Autodesk Inventor part; units mm, degrees
ref_plane "YZ Plane" through (0, 0, 0) normal (1, 0, 0) x (0, 1, 0)
ref_plane "XZ Plane" through (0, 0, 0) normal (0, 1, 0) x (-1, 0, 0)
ref_plane "XY Plane" through (0, 0, 0) normal (0, 0, 1) x (1, 0, 0)
sketch "Sketch1" plane through (0, 0, 0) normal (0, 0, 1) x (1, 0, 0)
  line L0 (0, 50.2073) -> (47.75, 15.5149) construction
  line L1 (47.75, 15.5149) -> (29.5111, -40.6186) construction
  line L2 (29.5111, -40.6186) -> (-29.5111, -40.6186) construction
  line L3 (-29.5111, -40.6186) -> (-47.75, 15.5149) construction
  line L4 (-47.75, 15.5149) -> (0, 50.2073) construction
  circle A0 centre (0, 50.2073) radius 4.5
  circle A1 centre (47.75, 15.5149) radius 4.5
  circle A2 centre (29.5111, -40.6186) radius 4.5
  circle A3 centre (-29.5111, -40.6186) radius 4.5
  circle A4 centre (-47.75, 15.5149) radius 4.5
  circle A5 centre (0, 0) radius 40
  circle A6 centre (0, 0) radius 60
  dimension "d0" = 95.5
  dimension "d1" = 9
  dimension "d2" = 80
  dimension "d3" = 120
extrude "Extrusion1" add sketch "Sketch1" along normal blind 50
properties part number "drive wheel sprocket spacer"
Work out the finished part from the listing and answer in its coordinate system (mm). Give positions to 0.01 mm unless a question says otherwise; leave off trailing zeros. Order: outer loops, then holes, each group sorted by start corner. A loop starts at its lowest first (then second) coordinate and runs counter-clockwise, first axis right, second up. Notation, with made-up numbers: (-38, -26.5) - (16, -26.5) arc R30 ccw to (16, 1.5) - close; hole circle Ø1 at (46.25, 15). An arc over 180 degrees is marked (long way). Answer as CSV lines item,"result". Start each with the question number.
Q1. The part is cut by section C-C (z = 44). Write down the section's boundary in (x, y), then the cut area to 3 significant figures.
Q2. The part is cut by section D-D (x = 13). Write down the section's boundary in (y, z), then the cut area to 3 significant figures.
Q3. The mould has two halves that part along Y. Classify faces 1 (the face through (-8.67, 39.05, 24.65)), 2 (the face through (-59.94, -2.64, 24.65)), 3 (the face through (39, -12, 0)): +Y half, -Y half, draft (parallel to the pull), parting line (faces both ways), or undercut.
Q4. Find the intervals of material crossed by L1, parallel to Y at x = 0, z = 39.5; L2, parallel to X at y = 13.5, z = 21; L3, parallel to Y at x = 31, z = 14, in increasing order. Write a range as [from, to].
Q5. Given pin 1 Ø1.5 at (x, z) = (45.5, 13.5) entering from -Y; pin 2 Ø12 at (x, z) = (-4, 42.5) entering from +Y; pin 3 Ø6 at (x, z) = (34, 23.5) entering from -Y, each flat-ended and moving along its own axis, determine where each tip first touches the part or whether it passes through.
Q6. The part is cut by section A-A (x = 0). Write down the section's boundary in (y, z), then the cut area to 3 significant figures.
Q7. The part is cut by section B-B (y = 0). Write down the section's boundary in (x, z), then the cut area to 3 significant figures.
Check result:
1,outline,"circle Ø120 at (0, 0); hole circle Ø9 at (-47.75, 15.51); hole circle Ø80 at (0, 0); hole circle Ø9 at (-29.51, -40.62); hole circle Ø9 at (0, 50.21); hole circle Ø9 at (29.51, -40.62); hole circle Ø9 at (47.75, 15.51)"
1,area,"5,970 mm²"
2,outline,"(-58.57, 0) - (-37.83, 0) - (-37.83, 50) - (-58.57, 50) - close; (37.83, 0) - (58.57, 0) - (58.57, 50) - (37.83, 50) - close"
2,area,"2,070 mm²"
3,face 1,"undercut"
3,face 2,"parting line"
3,face 3,"draft"
4,L1,"y = [-60, -40], [40, 45.71], [54.71, 60]"
4,L2,"x = [-58.46, -51.77], [-43.73, -37.65], [37.65, 43.73], [51.77, 58.46]"
4,L3,"y = [-51.37, -44.87], [-36.37, -25.28], [25.28, 51.37]"
5,pin 1,"stops at y = -39.97"
5,pin 2,"stops at y = 60"
5,pin 3,"stops at y = -51.37"
6,outline,"(-60, 0) - (-40, 0) - (-40, 50) - (-60, 50) - close; (40, 0) - (45.71, 0) - (45.71, 50) - (40, 50) - close; (54.71, 0) - (60, 0) - (60, 50) - (54.71, 50) - close"
6,area,"1,550 mm²"
7,outline,"(-60, 0) - (-40, 0) - (-40, 50) - (-60, 50) - close; (40, 0) - (60, 0) - (60, 50) - (40, 50) - close"
7,area,"2,000 mm²"
